Drawing for the job (mm, zero at the part's lowest x, y, z). A direction names the side the tool comes from. Round coordinates to 2 decimals unless told otherwise and drop trailing zeros. Order: outer loops, then holes, each group sorted by start corner. A loop starts at its lowest first (then second) coordinate and runs counter-clockwise, first axis right, second up. Notation, with made-up numbers: (4.25, -2) -> (48.25, -2) arc R17 cw to (48.25, 18) -> close; hole circle Ø6 at (-40, 78.5). An arc over 180 degrees is marked (long way). Use CSV: the item, a comma, the result in double quotes.
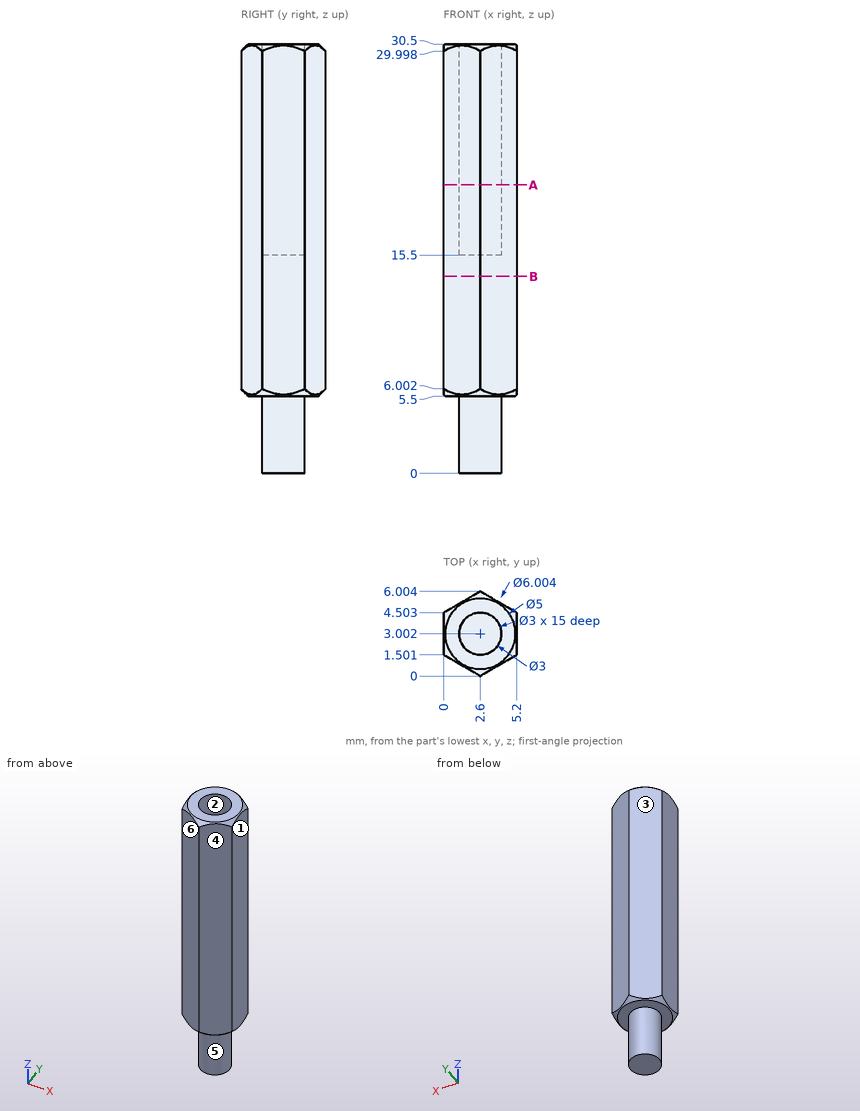
Q1. Pin check, flat tip, straight feed: pin 1 (2 mm diameter, centred on x = 3, z = 12.5, fed in from +Y). Stop position of the tip, or through.
From the geometry:
pin 1,"stops at y = 6"
Q2. Cut at A-A (z = 20.5). Give the cut face in (x, y) (1 decimal).
From the geometry:
outline,"(0, 1.5) -> (2.6, 0) -> (5.2, 1.5) -> (5.2, 4.5) -> (2.6, 6) -> (0, 4.5) -> close; hole circle Ø3 at (2.6, 3)"
Q3. Which spindle directions (+Z, -Z, +X, -X, +Y, -Y) get a long thin tool onto all of the face, cutting with end or side? Do the marked faces 5 and 6. Say none if no direction does.
From the geometry:
face 5,"-Z"
face 6,"+Z, -Z, -X, -Y"
Q4. Probe line 1 along Z through (x, y) = (0.45, 3.75); line 2 along Y through (x, z) = (1.9, 19) (1 decimal); line 3 along Z through (x, y) = (2.7, 4). List the from-to ranges inside material, lowest first.
From the geometry:
line 1,"z = 5.5 to 30.5"
line 2,"y = 0.4 to 1.7, 4.3 to 5.6"
line 3,"z = 0 to 15.5"
Q5. Cut at B-B (z = 14). Give the cut face in (x, y) (1 decimal).
From the geometry:
outline,"(0, 1.5) -> (2.6, 0) -> (5.2, 1.5) -> (5.2, 4.5) -> (2.6, 6) -> (0, 4.5) -> close"
Q6. Mould opens along Y. For the marked faces 1, 2, 3 and 4 say: +Y half, -Y half, draft (parallel to the pull), parting line (faces both ways), or undercut.
From the geometry:
face 1,"draft"
face 2,"undercut"
face 3,"+Y half"
face 4,"-Y half"
